Read the model definition and answer for the solid it produces. Units are mm, in the model's axes. Face numbers are marked on the shaded views. A direction names the side the tool comes from. Coordinates: 2 decimals unless noted, no trailing zeros.
from build123d import *

# Parameters (mm, degrees)
SKETCH_1_W      = 140
SKETCH_1_H      = 100
EXTRUDE_1_DEPTH = 10
EXTRUDE_2_DEPTH = 50
EXTRUDE_2_TAPER = 5


with BuildPart() as part:
    # 스케치1 → 보스-돌출1 (new body)
    with BuildSketch(Plane(origin=(0, 0, 0), x_dir=(1, 0, 0), z_dir=(0, 1, 0))):
        Rectangle(SKETCH_1_W, SKETCH_1_H)
    extrude(amount=EXTRUDE_1_DEPTH)

    # 스케치2 → 보스-돌출2 (add)
    with BuildSketch(Plane(origin=(0, 10, 0), x_dir=(1, 0, 0), z_dir=(0, 1, 0))):
        Polygon((20, 20), (20, 40), (-20, 40), (-20, 20), (-60, 20), (-60, -20), (-20, -20), (-20, -40), (20, -40), (20, -20), (60, -20), (60, 20), align=None)
    extrude(amount=EXTRUDE_2_DEPTH, taper=EXTRUDE_2_TAPER)


solid = part.part
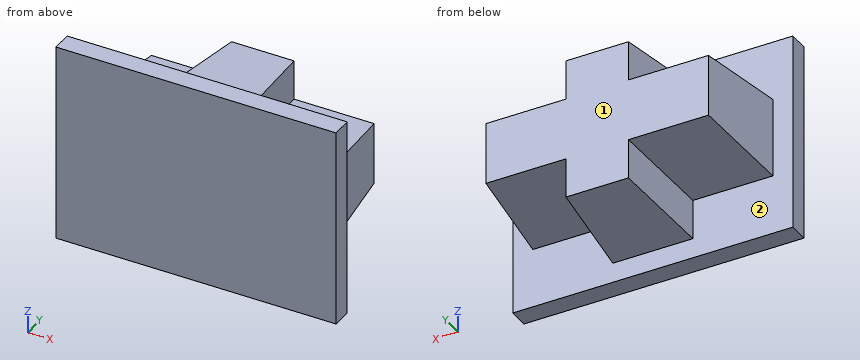
Q1. Straight lines are drawn through the part: probe 1 along Y at (x, z) = (31.5, -40); probe 2 along X at (y, z) = (30, 6.5); probe 3 along Z at (x, y) = (-42, 43). For each, find the intervals that lie inside material, in ascending order.
Findings below:
probe 1: y = 0 to 10
probe 2: x = -58.25 to 58.25
probe 3: z = -17.11 to 17.11
Q2. Which of the six approach directions +Z, -Z, +X, -X, +Y, -Y give full straight-line access (tool end or side, diameter ignored) to the marked faces 1 and 2?
Findings below:
face 1: +Z, -Z, +X, -X, +Y
face 2: +Y
Q3. Flat-ended cylindrical pins translate along their axes: pin 1 Ø1 at (y, z) = (46.5, -6.5) entering from +X; pin 2 Ø12 at (y, z) = (24, -23) entering from +X; pin 3 Ø12 at (x, y) = (36, 23) entering from -Z; pin 4 Ø12 at (y, z) = (11.5, 29.5) entering from +X. Find the tip coordinate at first contact, or state that the pin passes through.
Findings below:
pin 1: stops at x = 56.85
pin 2: stops at x = 59.18
pin 3: stops at z = -19.39
pin 4: stops at x = 70
